The listing builds one solid part. Answer for the finished solid, in the listing's coordinates (mm). Face numbers are marked on the shaded views. A direction names the side the tool comes from. Give positions to 0.01 mm unless a question says otherwise; leave off trailing zeros. Write each loop counter-clockwise with the first axis right and the second up, starting at its lowest first coordinate (ties: lowest second). Pieces come first, ordered by that corner, then holes. Notation, with made-up numbers: (-3, 24.5) - (8, 24.5) arc R12 cw to (8, 42.5) - close; hole circle Ø6 at (60.5, 78). An arc over 180 degrees is marked (long way). Write each question's results on one line, items separated by ' | '. Start each with the question number.
Q1. For a pull along Z with two mould halves and no side action, classify the marked faces 3, 4, 5 and 6 as pulls with the +Z half, pulls with the -Z half, needs draft (parallel to the pull), parting line crosses it, or undercut.
Q2. Section A-A (x = 68) is taken. Determine the outline of the cut face in (y, z).
Q3. Section B-B (z = -44) is taken. Determine the outline of the cut face in (x, y).
Q4. Section C-C (y = 66) is taken. Determine the outline of the cut face in (x, z), plus the area to 3 significant figures.
Q5. Find the intervals of material crossed by probe 1 along X at (y, z) = (14, 0); probe 2 along Z at (x, y) = (64, 119.5); probe 3 along Y at (x, z) = (45, 2.5), in increasing order.
Q6. For the marked faces 1 and 2, determine the directions among +Z, -Z, +X, -X, +Y, -Y from which every point of the face is accessible in a straight line to the end or side of a thin tool.
Q7. Flat-ended cylindrical pins translate along their axes: pin 1 Ø3 at (y, z) = (85, 11.5) entering from -X; pin 2 Ø12 at (x, y) = (67, 79.5) entering from +Z; pin 3 Ø10 at (y, z) = (15.5, -29) entering from +X; pin 4 Ø4 at (y, z) = (9, 1.5) entering from +X. Find the tip coordinate at first contact, or state that the pin passes through.
```python
from build123d import *

# Parameters (mm, degrees)
SKETCH1_R           = 50
BOSS_EXTRUDE1_DEPTH = 20
BOSS_EXTRUDE2_DEPTH = 150


with BuildPart() as part:
    # Sketch1 → Boss-Extrude1 (new body)
    with BuildSketch(Plane(origin=(0, 0, 0), x_dir=(1, 0, 0), z_dir=(0, 1, 0))):
        with BuildLine():
            ThreePointArc((50.339164764, 13.978703751), (-68.009745742, 0.022314378), (50.328751088, -14.02210054))
            Line((50.328751088, -14.02210054), (61.947059133, -14.02210054))
            Line((61.947059133, -14.02210054), (61.947059133, 13.978703751))
            Line((61.947059133, 13.978703751), (50.339164764, 13.978703751))
        make_face()
        with Locations((-8.009749891, 0)):
            Circle(SKETCH1_R, mode=Mode.SUBTRACT)
    extrude(amount=BOSS_EXTRUDE1_DEPTH)

    # Sketch1_4 → Boss-Extrude2 (add)
    with BuildSketch(Plane(origin=(0, 0, 0), x_dir=(1, 0, 0), z_dir=(0, 1, 0))):
        with BuildLine():
            Line((72.947059133, 3.978703751), (72.947059133, 0))
            Line((72.947059133, 0), (79.947059133, 0))
            ThreePointArc((79.947059133, 0), (79.617784148, 7.020172773), (78.632850446, 13.978703751))
            Line((78.632850446, 13.978703751), (61.947059133, 13.978703751))
            Line((61.947059133, 13.978703751), (61.947059133, 3.978703751))
            Line((61.947059133, 3.978703751), (72.947059133, 3.978703751))
        make_face()
        with BuildLine():
            Line((79.947059133, 0), (72.947059133, 0))
            Line((72.947059133, 0), (72.947059133, -4.02210054))
            Line((72.947059133, -4.02210054), (61.947059133, -4.02210054))
            Line((61.947059133, -4.02210054), (61.947059133, -14.02210054))
            Line((61.947059133, -14.02210054), (78.624604535, -14.02210054))
            ThreePointArc((78.624604535, -14.02210054), (79.615713551, -7.042162127), (79.947059133, 0))
        make_face()
    extrude(amount=BOSS_EXTRUDE2_DEPTH)


solid = part.part
```
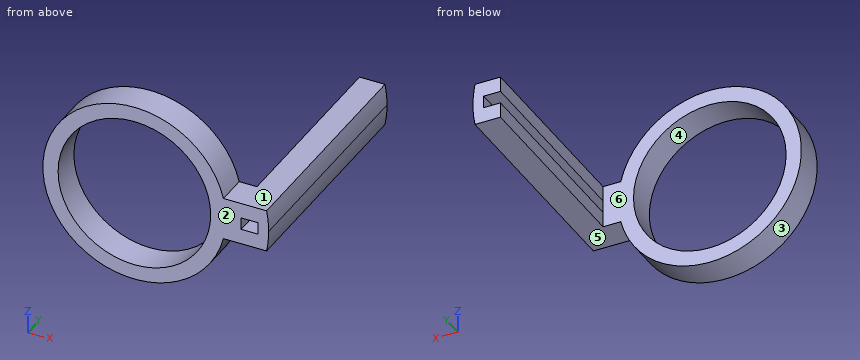
Answers below:
1) face 3: parting line crosses it | face 4: undercut | face 5: pulls with the -Z half | face 6: needs draft
2) outline: (0, -13.98) - (150, -13.98) - (150, -3.98) - (0, -3.98) - close; (0, 4.02) - (150, 4.02) - (150, 14.02) - (0, 14.02) - close
3) outline: (-48.8, 0) - (-31.76, 0) - (-31.76, 20) - (-48.8, 20) - close; (15.74, 0) - (32.78, 0) - (32.78, 20) - (15.74, 20) - close
4) outline: (61.95, -13.98) - (78.63, -13.98) arc R75 ccw to (78.62, 14.02) - (61.95, 14.02) - (61.95, 4.02) - (72.95, 4.02) - (72.95, -3.98) - (61.95, -3.98) - close | area: 404 mm2
5) probe 1: x = -68.01 to -58.01, 41.99 to 61.95, 72.95 to 79.95 | probe 2: z = -13.98 to -3.98, 4.02 to 14.02 | probe 3: y = 0 to 20
6) face 1: +Z, +X, +Y, -Y | face 2: +Z, -Z, +X, -X, -Y
7) pin 1: stops at x = 61.95 | pin 2: stops at z = 14.02 | pin 3: stops at x = 46.98 | pin 4: stops at x = 79.95
